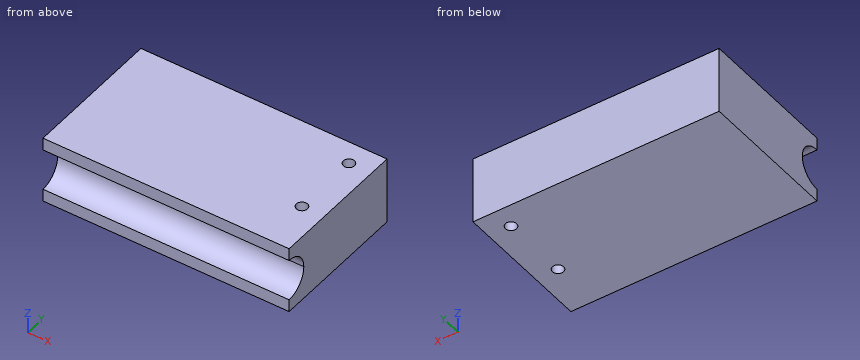
from build123d import *

# Parameters (mm, degrees)
F0_W     = 139.7
F0_H     = 79.375
F0_R     = 3.175
F1_DEPTH = 38.1
F3_DEPTH = 139.701


with BuildPart() as f1:
    # F0 (on Top) → F1 (new body)
    with BuildSketch(Plane.XY):
        Rectangle(F0_W, F0_H)
        with Locations((57.15, -11.1125)):
            Circle(F0_R, mode=Mode.SUBTRACT)
        with Locations((57.15, 26.9875)):
            Circle(F0_R, mode=Mode.SUBTRACT)
    extrude(amount=F1_DEPTH)

    # F2 (on face) → F3 (cut, through all)
    with BuildSketch(Plane.YZ.offset(69.85)):
        with BuildLine():
            ThreePointArc((-39.6875, 7.1374), (-31.26402, 10.62652), (-27.7749, 19.05))
            ThreePointArc((-27.7749, 19.05), (-31.26402, 27.47348), (-39.6875, 30.9626))
            Line((-39.6875, 30.9626), (-39.6875, 7.1374))
        make_face()
    extrude(amount=-F3_DEPTH, mode=Mode.SUBTRACT)


solid = f1.part
Model file for the job. Use its own axes, mm. Coordinates: 2 decimals unless noted, no trailing zeros. Order: outer loops, then holes, each group sorted by start corner. A loop starts at its lowest first (then second) coordinate and runs counter-clockwise, first axis right, second up. Notation, with made-up numbers: (51, 65) -> (82, 65) arc R12 ccw to (82, 69) -> close; hole circle Ø1 at (86, 7.5). An arc over 180 degrees is marked (long way). Return JSON: item names as keys, results as strings. Group by question number.
Item 1: Wall check: line 1 along X through (y, z) = (-11, 36); line 2 along Y through (x, z) = (57, 18); line 3 along Y through (x, z) = (54.5, 22). Give the ranges that are in metal, low to high. Write a range as [from, to].
Item 2: Saw through at A-A on x = 57.15. Write the cut outline in (y, z), then the cut area to 3 significant figures.
Item 3: Saw through at D-D on z = 21. State how many separate pieces and enclosed holes the cut face has, then the cut area to 3 significant figures.
Item 4: Saw through at C-C on x = -40. Write the cut outline in (y, z), then the cut area to 3 significant figures.
Item 5: Saw through at B-B on y = -31. Write the cut outline in (x, z), then the cut area to 3 significant figures.
Values found:
{
 "1": {"line 1": "x = [-69.85, 53.98], [60.32, 69.85]", "line 2": "y = [-27.82, -14.28], [-7.94, 23.82], [30.16, 39.69]", "line 3": "y = [-28.15, -12.86], [-9.36, 25.24], [28.74, 39.69]"},
 "2": {"outline": "(-39.69, 0) -> (-14.29, 0) -> (-14.29, 38.1) -> (-39.69, 38.1) -> (-39.69, 30.96) arc R11.91 cw to (-27.77, 19.05) arc R11.91 cw to (-39.69, 7.14) -> close; (-7.94, 0) -> (23.81, 0) -> (23.81, 38.1) -> (-7.94, 38.1) -> close; (30.16, 0) -> (39.69, 0) -> (39.69, 38.1) -> (30.16, 38.1) -> close", "area": "2,320 mm2"},
 "3": {"separate pieces": "1", "enclosed holes": "2", "area": "9,380 mm2"},
 "4": {"outline": "(-39.69, 0) -> (39.69, 0) -> (39.69, 38.1) -> (-39.69, 38.1) -> (-39.69, 30.96) arc R11.91 cw to (-27.77, 19.05) arc R11.91 cw to (-39.69, 7.14) -> close", "area": "2,800 mm2"},
 "5": {"outline": "(-69.85, 0) -> (69.85, 0) -> (69.85, 10.9) -> (-69.85, 10.9) -> close; (-69.85, 27.2) -> (69.85, 27.2) -> (69.85, 38.1) -> (-69.85, 38.1) -> close", "area": "3,050 mm2"}
}
